Can you work these out from the model? Positions are in its coordinate system, mm. A direction names the side the tool comes from. Give positions to 0.01 mm unless a question says otherwise; leave off trailing zeros. Order: outer loops, then holes, each group sorted by start corner. A loop starts at its lowest first (then second) coordinate and runs counter-clockwise, first axis right, second up.
Item 1: I want a section at D-D, the plane z = -54. Write out the boundary of the cut face in (x, y).
Item 2: I want a section at C-C, the plane x = -162.68. Write out the boundary of the cut face in (y, z) (3 decimals), then the cut area to 3 significant figures.
Item 3: I want a section at B-B, the plane z = -11.5. Write out the boundary of the cut face in (x, y), then the cut area to 3 significant figures.
Item 4: If we mould it in two halves opening along Y, with no side actions, what happens to faces 6 (the flat face through (-145, -8, -22.57)), 7 (the flat face through (-77.76, -2.83, -35.76)), 8 (the flat face through (-128.4, 1.9, -24.59)), 9 (the cylindrical face through (-179.39, -2.17, -29.1))? For each: +Y half, -Y half, draft (parallel to the pull), parting line (faces both ways), or undercut.
Item 5: I'm going to push flat-ended pins straight in: pin 1 Ø6 at (x, y) = (-157.5, -8.5) entering from +Z; pin 2 Ø5 at (y, z) = (-8.51, -26.285) entering from -X; pin 3 Ø8 at (x, y) = (-169, 16) entering from -Z. Where does each tip first touch, or does it pass through?
Item 6: I want a section at A-A, the plane x = -127.33. Write out the boundary of the cut face in (y, z) (3 decimals).
Item 7: Which directions (+Z, -Z, +X, -X, +Y, -Y) give clear straight access to the entire face, cutting with the end or side of a thin tool? Please do faces 1 (the flat face through (-96, 21.25, -30)), 2 (the flat face through (-180.25, 0, -15)), 3 (the flat face through (-119.75, -3, -45)), 4 (the flat face through (-87, 24, -49.66)), 5 (the cylindrical face through (-131.995, -23.064, -20.235)).
Item 8: If I drill on line 1 along Y through (x, z) = (-145, -19.25); line 2 along X through (y, z) = (-7.5, -14); line 3 along X through (y, z) = (4, -23), over which ranges is the centre line in solid material (lowest first)?
```python
from build123d import *

# Parameters (mm, degrees)
CROQUIS1_W              = 65.5
CROQUIS1_H              = 52.5
SALIENTE_EXTRUIR1_DEPTH = 30
CROQUIS2_W              = 60.8
CROQUIS2_H              = 42.1
CORTAR_EXTRUIR1_DEPTH   = 16
CROQUIS3_W              = 5
CROQUIS3_H              = 52.5
SALIENTE_EXTRUIR2_DEPTH = 30
CROQUIS4_W              = 60
CROQUIS4_H              = 5
SALIENTE_EXTRUIR3_DEPTH = 30
CROQUIS5_R              = 10.1
CORTAR_EXTRUIR2_DEPTH   = 6.57
CROQUIS7_R              = 5.05
CORTAR_EXTRUIR3_DEPTH   = 8.59
CROQUIS8_R              = 2.275
CORTAR_EXTRUIR4_DEPTH   = 8.59
CROQUIS9_W              = 60.5
CROQUIS9_H              = 30
SALIENTE_EXTRUIR4_DEPTH = 5
CORTAR_EXTRUIR5_DEPTH   = 5
CROQUIS11_W             = 41
CROQUIS11_H             = 60
SALIENTE_EXTRUIR5_DEPTH = 5
CROQUIS12_W             = 5
CROQUIS12_H             = 60
SALIENTE_EXTRUIR6_DEPTH = 47.5
CROQUIS13_W             = 18
CROQUIS13_H             = 10.34
CORTAR_EXTRUIR6_DEPTH   = 10
CROQUIS14_W             = 17.194416488
CROQUIS14_H             = 64.089157204
CORTAR_EXTRUIR7_DEPTH   = 10
CORTAR_EXTRUIR8_DEPTH   = 10
REDONDEO1_R             = 3
REDONDEO6_R             = 3
REDONDEO7_R             = 3
CAVIDAD1_START          = -32.75
CAVIDAD1_DEPTH          = 5
CROQUIS16_R             = 1.5
CORTAR_EXTRUIR10_DEPTH  = 10
CAVIDAD3_START          = -73.75
CAVIDAD3_OUTLINE_R      = 1.515
CAVIDAD3_DEPTH          = 106.5
CROQUIS17_R             = 3
CORTAR_EXTRUIR11_DEPTH  = 5
REDONDEO8_R             = 3
REDONDEO9_R             = 3


# Read off the part's stored shape, not the designer's step: Cavidad1, Cavidad3
with BuildPart() as part:
    # Croquis1 → Saliente-Extruir1 (new body)
    with BuildSketch(Plane.XY):
        Rectangle(CROQUIS1_W, CROQUIS1_H)
    extrude(amount=-SALIENTE_EXTRUIR1_DEPTH)

    # Croquis2 → Cortar-Extruir1 (cut)
    with BuildSketch(Plane.XY):
        with Locations((-2.35, -5.2)):
            Rectangle(CROQUIS2_W, CROQUIS2_H)
    extrude(amount=-CORTAR_EXTRUIR1_DEPTH, mode=Mode.SUBTRACT)

    # Croquis3 → Saliente-Extruir2 (add)
    with BuildSketch(Plane(origin=(0, 0, -30), x_dir=(-1, 0, 0), z_dir=(0, 0, -1))):
        with Locations((30.25, 0)):
            Rectangle(CROQUIS3_W, CROQUIS3_H)
    extrude(amount=SALIENTE_EXTRUIR2_DEPTH)

    # Croquis4 → Saliente-Extruir3 (add)
    with BuildSketch(Plane.ZY.offset(32.75)):
        with Locations((-30, 23.75)):
            Rectangle(CROQUIS4_W, CROQUIS4_H)
    extrude(amount=SALIENTE_EXTRUIR3_DEPTH)

    # Croquis5 → Cortar-Extruir2 (cut)
    with BuildSketch(Plane.XY.offset(-16)):
        with Locations((-2.5, -8.51)):
            Circle(CROQUIS5_R)
    extrude(amount=-CORTAR_EXTRUIR2_DEPTH, mode=Mode.SUBTRACT)

    # Croquis7 → Cortar-Extruir3 (cut)
    with BuildSketch(Plane.XY.offset(-16)):
        with Locations((-20.17, 4.12)):
            Circle(CROQUIS7_R)
        with Locations((15.18, 4.12)):
            Circle(CROQUIS7_R)
        with Locations((15.18, -21.13)):
            Circle(CROQUIS7_R)
        with Locations((-20.17, -21.13)):
            Circle(CROQUIS7_R)
    extrude(amount=-CORTAR_EXTRUIR3_DEPTH, mode=Mode.SUBTRACT)

    # Croquis8 → Cortar-Extruir4 (cut)
    with BuildSketch(Plane.XY.offset(-24.59)):
        with Locations((-20.17, 4.12)):
            Circle(CROQUIS8_R)
        with Locations((-20.17, -21.13)):
            Circle(CROQUIS8_R)
        with Locations((15.18, 4.12)):
            Circle(CROQUIS8_R)
        with Locations((15.18, -21.13)):
            Circle(CROQUIS8_R)
    extrude(amount=-CORTAR_EXTRUIR4_DEPTH, mode=Mode.SUBTRACT)

    # Croquis9 → Saliente-Extruir4 (add)
    with BuildSketch(Plane(origin=(0, 26.25, 0), x_dir=(1, 0, 0), z_dir=(0, 1, 0))):
        with Locations((2.5, 45)):
            Rectangle(CROQUIS9_W, CROQUIS9_H)
    extrude(amount=-SALIENTE_EXTRUIR4_DEPTH)

    # Croquis10 → Cortar-Extruir5 (cut)
    with BuildSketch(Plane.XZ.offset(-21.25)):
        Polygon((32.75, -30), (-27.75, -60), (-30.096630242, -66.962952029), (62.11742193, -82.705107475), (54.436655983, -30), align=None)
    extrude(amount=-CORTAR_EXTRUIR5_DEPTH, mode=Mode.SUBTRACT)

    # Croquis11 → Saliente-Extruir5 (add)
    with BuildSketch(Plane.XZ.offset(-21.25)):
        with Locations((-53.25, -30)):
            Rectangle(CROQUIS11_W, CROQUIS11_H)
    extrude(amount=-SALIENTE_EXTRUIR5_DEPTH)

    # Croquis12 → Saliente-Extruir6 (add)
    with BuildSketch(Plane.XZ.offset(-21.25)):
        with Locations((-71.25, -30)):
            Rectangle(CROQUIS12_W, CROQUIS12_H)
    extrude(amount=SALIENTE_EXTRUIR6_DEPTH)

    # Croquis13 → Cortar-Extruir6 (cut)
    with BuildSketch(Plane.XZ.offset(-21.25)):
        with Locations((-59.75, -54.83)):
            Rectangle(CROQUIS13_W, CROQUIS13_H)
    extrude(amount=-CORTAR_EXTRUIR6_DEPTH, mode=Mode.SUBTRACT)

    # Croquis14 → Cortar-Extruir7 (cut)
    with BuildSketch(Plane(origin=(-68.75, 0, 0), x_dir=(0, 0, -1), z_dir=(1, 0, 0))):
        with Locations((58.257208244, -5.794578602)):
            Rectangle(CROQUIS14_W, CROQUIS14_H)
    extrude(amount=-CORTAR_EXTRUIR7_DEPTH, mode=Mode.SUBTRACT)

    # Croquis15 → Cortar-Extruir8 (cut)
    with BuildSketch(Plane(origin=(-68.75, 0, 0), x_dir=(0, 0, -1), z_dir=(1, 0, 0))):
        Polygon((15.02, -38.75), (49.66, 21.25), (49.66, -38.75), align=None)
    extrude(amount=-CORTAR_EXTRUIR8_DEPTH, mode=Mode.SUBTRACT)

    # Redondeo1
    redondeo1_edges = [part.edges().sort_by_distance(p)[0] for p in [
        (32.75, 0, 0),
    ]]
    fillet(redondeo1_edges, radius=REDONDEO1_R)

    # Redondeo6
    redondeo6_edges = [part.edges().sort_by_distance(p)[0] for p in [
        (32.75, -2.5, -30),
    ]]
    fillet(redondeo6_edges, radius=REDONDEO6_R)

    # Redondeo7
    redondeo7_edges = [part.edges().sort_by_distance(p)[0] for p in [
        (32.75, 23.75, -30),
    ]]
    fillet(redondeo7_edges, radius=REDONDEO7_R)

    # Cavidad1 outline → Cavidad1 (cut)
    with BuildSketch(Plane.YZ.offset(CAVIDAD1_START)):
        with BuildLine():
            ThreePointArc((5.82457056, -60), (-8.75, -50.820508076), (-23.32457056, -60))
            Line((-23.32457056, -60), (5.82457056, -60))
        make_face()
    extrude(amount=CAVIDAD1_DEPTH, mode=Mode.SUBTRACT)

    # Croquis16 → Cortar-Extruir10 (cut)
    with BuildSketch(Plane.ZY.offset(-28.05)):
        with Locations((-26.285, -8.51)):
            Circle(CROQUIS16_R)
    extrude(amount=-CORTAR_EXTRUIR10_DEPTH, mode=Mode.SUBTRACT)

    # Cavidad3 outline → Cavidad3 (cut)
    with BuildSketch(Plane.YZ.offset(CAVIDAD3_START)):
        with Locations((-8.51, -26.285)):
            Circle(CAVIDAD3_OUTLINE_R)
    extrude(amount=CAVIDAD3_DEPTH, mode=Mode.SUBTRACT)

    # Croquis17 → Cortar-Extruir11 (cut)
    with BuildSketch(Plane(origin=(32.75, 0, 0), x_dir=(0, 0, -1), z_dir=(1, 0, 0))):
        with Locations(Location((26.285, -8.51, 0), (0, 0, 90))):
            Circle(CROQUIS17_R)
    extrude(amount=-CORTAR_EXTRUIR11_DEPTH, mode=Mode.SUBTRACT)

    # Redondeo8
    redondeo8_edges = [part.edges().sort_by_distance(p)[0] for p in [
        (-73.75, 0, 0),
    ]]
    fillet(redondeo8_edges, radius=REDONDEO8_R)

    # Redondeo9
    redondeo9_edges = [part.edges().sort_by_distance(p)[0] for p in [
        (-73.75, 23.75, -49.66),
        (-73.75, -2.5, -35.948333333),
    ]]
    fillet(redondeo9_edges, radius=REDONDEO9_R)


with BuildPart() as body_2:
    # Simetría1: mirrored copy
    add(part.part.mirror(Plane(origin=(-73.75, 26.25, 0), x_dir=(0, 0, 1), z_dir=(-1, 0, 0))))


solid = body_2.part
```
Results list:
1. outline: (-131.85, 21.25) - (-119.75, 21.25) - (-119.75, 0.88) - (-114.75, 0.88) - (-114.75, 21.25) - (-96.75, 21.25) - (-96.75, 26.25) - (-131.85, 26.25) - close; (-119.75, -26.25) - (-114.75, -26.25) - (-114.75, -18.38) - (-119.75, -18.38) - close
2. outline: (-26.25, -30) - (-23.405, -30) - (-23.405, -24.59) - (-26.18, -24.59) - (-26.18, -16) - (-26.25, -16) - close; (-18.855, -30) - (1.845, -30) - (1.845, -24.59) - (-0.93, -24.59) - (-0.93, -16) - (-16.08, -16) - (-16.08, -24.59) - (-18.855, -24.59) - close; (6.395, -30) - (21.25, -30) - (21.25, -38.712) - (26.25, -38.712) - (26.25, 0) - (15.85, 0) - (15.85, -16) - (9.17, -16) - (9.17, -24.59) - (6.395, -24.59) - close; hole circle Ø3.03 at (-8.51, -26.285)
2. area: 715 mm2
3. outline: (-180.25, -26.25) - (-175.55, -26.25) - (-175.55, 15.85) - (-114.75, 15.85) - (-114.75, 21.25) - (-78.75, 21.25) - (-78.75, -26.25) - (-73.75, -26.25) - (-73.75, 26.25) - (-180.25, 26.25) - close
3. area: 1,320 mm2
4. face 6: undercut
4. face 7: -Y half
4. face 8: undercut
4. face 9: draft
5. pin 1: stops at z = -16
5. pin 2: stops at x = -175.25
5. pin 3: stops at z = -30
6. outline: (-26.25, -30) - (-23.405, -30) - (-23.405, -24.59) - (-26.18, -24.59) - (-26.18, -16) - (-26.25, -16) - close; (-18.855, -30) - (1.845, -30) - (1.845, -24.59) - (-0.93, -24.59) - (-0.93, -16) - (-16.08, -16) - (-16.08, -24.59) - (-18.855, -24.59) - close; (6.395, -30) - (21.25, -30) - (21.25, -56.241) - (26.25, -56.241) - (26.25, 0) - (15.85, 0) - (15.85, -16) - (9.17, -16) - (9.17, -24.59) - (6.395, -24.59) - close; hole circle Ø3.03 at (-8.51, -26.285)
7. face 1: +Z, -Z, -Y
7. face 2: +Z, -Z, -X, +Y, -Y
7. face 3: -Z, -X, -Y
7. face 4: -Z, +X, +Y, -Y
7. face 5: +Z
8. line 1: y = -26.25 to -18.61, 1.59 to 26.25
8. line 2: x = -180.25 to -175.55, -78.75 to -73.75
8. line 3: x = -180.25 to -167.73, -157.63 to -132.38, -122.28 to -114.75, -78.75 to -73.75
